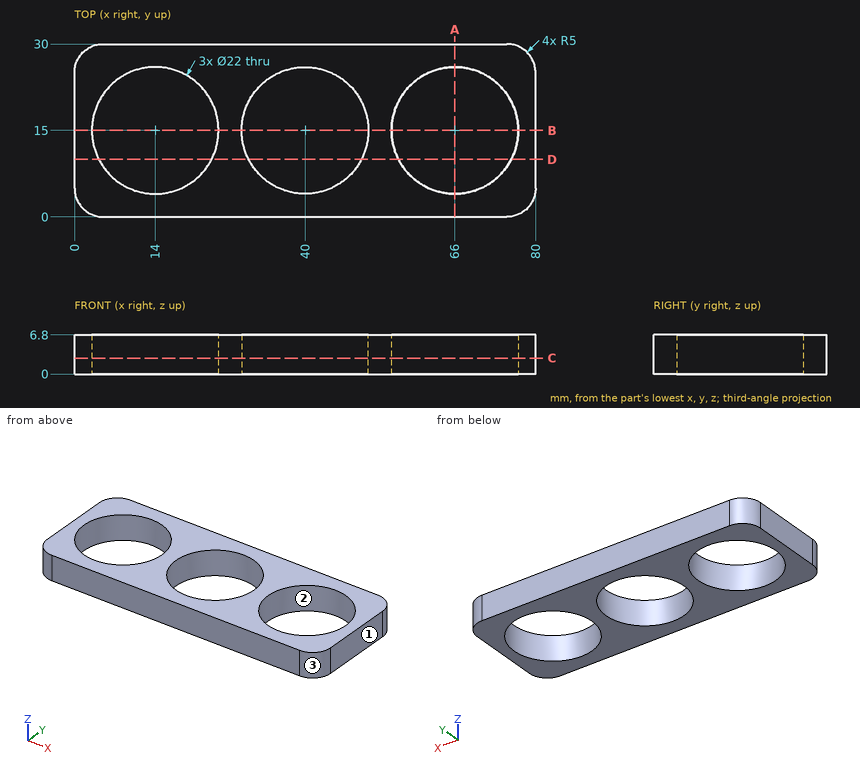
Input: dimensioned drawing with shaded views. Units: mm. Origin: part minimum x, y, z. Give positions to 0.01 mm unless a question says otherwise; leave off trailing zeros. Write each loop counter-clockwise with the first axis right and the second up, starting at its lowest first coordinate (ties: lowest second). Pieces come first, ordered by that corner, then holes. Notation, with made-up numbers: (83, -27.75) - (93, -27.75) arc R25 ccw to (93, -11.75) - close; hole circle Ø10 at (22, 13.25). An arc over 180 degrees is marked (long way). Write item = value, one per line. Start each with the question number.
1) Material intervals for L1, parallel to Y at x = 66, z = 3.25; L2, parallel to X at y = 6, z = 6; L3, parallel to Y at x = 56, z = 5.75, sorted ascending. Write a range as [from, to].
2) Draft query along Y for the marked faces 1, 2 and 3. Return one class per face: pulls with the +Y half, pulls with the -Y half, needs draft (parallel to the pull), parting line crosses it, or undercut.
3) Cut plane C-C (z = 2.75). Return loops of the section in (x, y).
4) Cut plane B-B (y = 15). Return loops of the section in (x, z), and give its area (3 significant figures).
5) Cut plane A-A (x = 66). Return loops of the section in (y, z).
6) Cut plane D-D (y = 10). Return loops of the section in (x, z).
Answers follow:
q1.L1 = [0, 4], [26, 30]
q1.L2 = [0, 7.68], [20.32, 33.68], [46.32, 59.68], [72.32, 80]
q1.L3 = [0, 10.42], [19.58, 30]
q2.face_1 = needs draft
q2.face_2 = undercut
q2.face_3 = pulls with the -Y half
q3.outline = (0, 5) arc R5 ccw to (5, 0) - (75, 0) arc R5 ccw to (80, 5) - (80, 25) arc R5 ccw to (75, 30) - (5, 30) arc R5 ccw to (0, 25) - close; hole circle Ø22 at (14, 15); hole circle Ø22 at (40, 15); hole circle Ø22 at (66, 15)
q4.outline = (0, 0) - (3, 0) - (3, 6.8) - (0, 6.8) - close; (25, 0) - (29, 0) - (29, 6.8) - (25, 6.8) - close; (51, 0) - (55, 0) - (55, 6.8) - (51, 6.8) - close; (77, 0) - (80, 0) - (80, 6.8) - (77, 6.8) - close
q4.area = 95.2 mm^2
q5.outline = (0, 0) - (4, 0) - (4, 6.8) - (0, 6.8) - close; (26, 0) - (30, 0) - (30, 6.8) - (26, 6.8) - close
q6.outline = (0, 0) - (4.2, 0) - (4.2, 6.8) - (0, 6.8) - close; (23.8, 0) - (30.2, 0) - (30.2, 6.8) - (23.8, 6.8) - close; (49.8, 0) - (56.2, 0) - (56.2, 6.8) - (49.8, 6.8) - close; (75.8, 0) - (80, 0) - (80, 6.8) - (75.8, 6.8) - close
